Read the model definition and answer for the solid it produces. Units are mm, in the model's axes. Round coordinates to 2 decimals unless told otherwise and drop trailing zeros. Order: outer loops, then holes, each group sorted by start corner. A loop starts at its lowest first (then second) coordinate and runs counter-clockwise, first axis right, second up. Notation, with made-up numbers: (46, 6.25) - (86, 6.25) arc R11 cw to (86, 15.25) - close; hole circle Ø7 at (-7.75, 60). An arc over 180 degrees is marked (long way). Answer as a JSON object with one key per item and string values. Group by question number.
Q1. A cutting plane is placed at A-A on x = 50.8. Determine the outline of the cut face in (y, z) (3 decimals), and give its area (3 significant figures).
Q2. A cutting plane is placed at C-C on z = 4.75. Count the separate pieces of the cut face and the enclosed holes in it, and give its area (3 significant figures).
Q3. A cutting plane is placed at D-D on x = 207. Determine the outline of the cut face in (y, z) (3 decimals), and give its area (3 significant figures).
Q4. A cutting plane is placed at B-B on y = 32. Determine the outline of the cut face in (x, z), and give its area (3 significant figures).
Q5. Given pin 1 Ø22.5 at (x, y) = (127, 19.05) entering from +Z, flat-ended and moving along its own axis, determine where the tip first touches the part or whether it passes through.
Q6. Consider line 1 (X direction, y = 36, z = 5.75); line 2 (X direction, y = 2, z = 3.5) (3 decimals); line 3 (X direction, y = 20, z = 0.5). Determine where each line is inside the solid, lowest interval first.
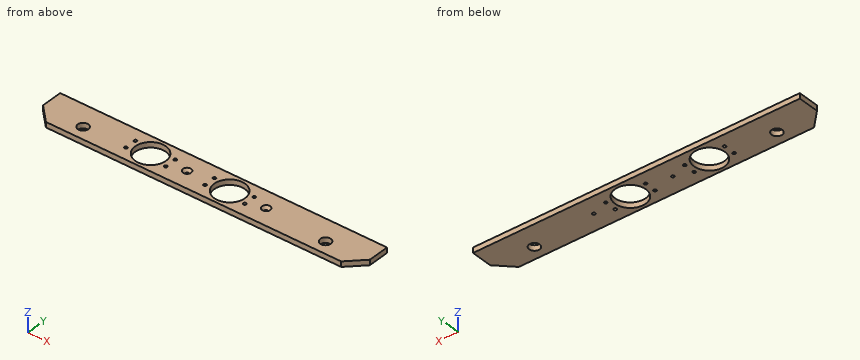
Autodesk Inventor part; units mm, degrees
ref_plane "YZ Plane" through (0, 0, 0) normal (1, 0, 0) x (0, 1, 0)
ref_plane "XZ Plane" through (0, 0, 0) normal (0, 1, 0) x (-1, 0, 0)
ref_plane "XY Plane" through (0, 0, 0) normal (0, 0, 1) x (1, 0, 0)
sketch "Sketch1" plane through (0, 0, 0) normal (0, 0, 1) x (1, 0, 0)
  circle A0 centre (127, 19.05) radius 18.542
  circle A1 centre (222.25, 19.05) radius 18.542
  circle A2 centre (170.942, 19.05) radius 1.778
  circle A3 centre (266.192, 19.05) radius 1.778
  line L0 (151.003, 19.05) -> (151.003, 26.0604)
  circle A4 centre (102.997, 12.0396) radius 1.7526
  circle A5 centre (102.997, 26.0604) radius 1.7526
  circle A6 centre (151.003, 26.0604) radius 1.7526
  circle A7 centre (151.003, 12.0396) radius 1.7526
  line L1 (151.003, 19.05) -> (127, 19.05)
  circle A8 centre (246.253, 26.0604) radius 1.7526
  circle A9 centre (246.253, 12.0396) radius 1.7526
  circle A10 centre (198.247, 12.0396) radius 1.7526
  circle A11 centre (198.247, 26.0604) radius 1.7526
  line L2 (0, -3.175) -> (393.7, -3.175)
  line L3 (0, 41.275) -> (393.7, 41.275)
  line L4 (0, 41.275) -> (0, -3.175)
  line L5 (393.7, 41.275) -> (393.7, -3.175)
  circle A12 centre (222.25, 19.05) radius 18.542
  circle A13 centre (246.253, 26.0604) radius 1.7526
  circle A14 centre (246.253, 12.0396) radius 1.7526
  circle A15 centre (266.192, 19.05) radius 1.778
  circle A16 centre (198.247, 12.0396) radius 1.7526
  circle A17 centre (198.247, 26.0604) radius 1.7526
  circle A18 centre (170.942, 19.05) radius 1.778
  circle A19 centre (151.003, 12.0396) radius 1.7526
  circle A20 centre (151.003, 26.0604) radius 1.7526
  circle A21 centre (127, 19.05) radius 18.542
  circle A22 centre (102.997, 12.0396) radius 1.7526
  circle A23 centre (102.997, 26.0604) radius 1.7526
  circle A24 centre (50.8, 12.7) radius 6.35
  circle A25 centre (342.9, 12.7) radius 6.35
  point P0 (0, 0)
  dimension "d3" = 37.084
  dimension "d5" = 37.084
  dimension "d10" = 3.556
  dimension "d11" = 3.556
  dimension "d24" = 7.0104
  dimension "d28" = 3.5052
  dimension "d29" = 3.5052
  dimension "d30" = 3.5052
  dimension "d31" = 24.003
  dimension "d38" = 3.5052
  dimension "d39" = 3.5052
  dimension "d40" = 3.5052
  dimension "d41" = 3.5052
extrude "Extrusion4" add sketch "Sketch1" along normal blind 6.35 contours L4 L3 L5 L2 | A24 | A25
chamfer "Chamfer2" distance 3.175 angle 45 2 edges at (169.164, 19.05, 6.35) (264.414, 19.05, 6.35)
extrude "Extrusion5" cut sketch "Sketch1" along normal blind 25.4 contours A24 | A25
chamfer "Chamfer3" distance 19.05 angle 45 1 edges at (0, -3.175, 3.175)
chamfer "Chamfer4" distance 19.05 angle 45 1 edges at (393.7, -3.175, 3.175)
properties part number "Drive Train - Smallest Model"
Result set:
{
 "1": {"outline": "(-3.175, 0) - (6.35, 0) - (6.35, 6.35) - (-3.175, 6.35) - close; (19.05, 0) - (41.275, 0) - (41.275, 6.35) - (19.05, 6.35) - close", "area": "202 mm²"},
 "2": {"separate pieces": "1", "enclosed holes": "14", "area": "14,600 mm²"},
 "3": {"outline": "(-3.175, 0) - (8.503, 0) - (8.503, 6.35) - (-3.175, 6.35) - close; (29.597, 0) - (41.275, 0) - (41.275, 6.35) - (29.597, 6.35) - close", "area": "148 mm²"},
 "4": {"outline": "(0, 0) - (113.73, 0) - (113.73, 6.35) - (0, 6.35) - close; (140.27, 0) - (208.98, 0) - (208.98, 6.35) - (140.27, 6.35) - close; (235.52, 0) - (393.7, 0) - (393.7, 6.35) - (235.52, 6.35) - close", "area": "2,160 mm²"},
 "5": {"pin 1": "passes through"},
 "6": {"line 1": "x = 0 to 119.48, 134.52 to 214.73, 229.77 to 393.7", "line 2": "x = 13.875 to 119.713, 134.287 to 214.963, 229.537 to 379.825", "line 3": "x = 0 to 108.48, 145.52 to 169.44, 172.44 to 203.73, 240.77 to 264.69, 267.69 to 393.7"}
}
